Read the model definition and answer for the solid it produces. Units are mm, in the model's axes. Face numbers are marked on the shaded views. Give positions to 0.01 mm unless a question says otherwise; leave off trailing zeros. Order: outer loops, then holes, each group sorted by start corner. A loop starts at its lowest first (then second) coordinate and runs counter-clockwise, first axis right, second up. Notation, with made-up numbers: (80, 78.5) - (133, 78.5) arc R12 ccw to (133, 87.5) - close; hole circle Ø2 at (74.25, 38.5). An arc over 180 degrees is marked (long way). Write each question's results on one line, items separated by ' | '. Start each with the question number.
Q1. Flat-ended cylindrical pins translate along their axes: P1, Ø2.5, axis at x = 42, y = 40.5, coming from the +Z side; P2, Ø6, axis at x = -41, y = 41, coming from the +Z side; P3, Ø10.5, axis at x = 41, y = -41, coming from the +Z side; P4, Ø12, axis at x = -57.98, y = 0, coming from the -Z side. Find the tip coordinate at first contact, or state that the pin passes through.
Q2. Find section B-B on z = 4.25. Give the vertices of the cut face in (x, y).
Q3. Find the intervals of material crossed by line 1 along Y through (x, z) = (0, 8); line 2 along Y through (x, z) = (39, 15); line 3 along Z through (x, y) = (20, 31), in increasing order. Write a range as from..to.
Q4. For a pull along Y with two mould halves and no side action, classify the marked faces 1 and 2 as +Y half, -Y half, draft (parallel to the pull), parting line (faces both ways), or undercut.
Q5. Find section C-C on x = 115. Give the vertices of the cut face in (y, z).
Q6. Find section D-D on y = 83. Give the vertices of the cut face in (x, z).
Q7. Find section A-A on y = 0. Give the vertices of the cut face in (x, z), and give its area (3 significant figures).
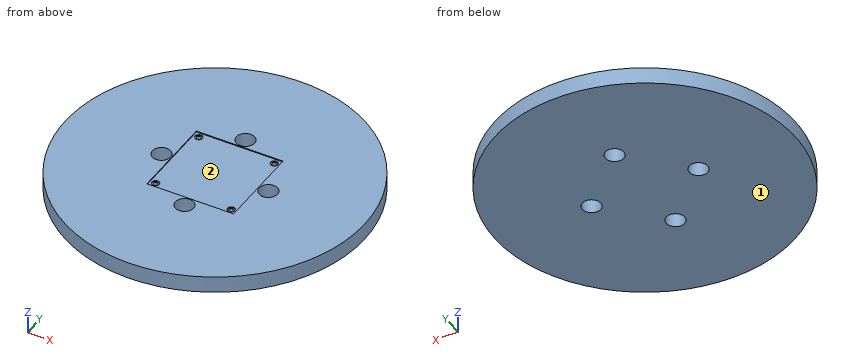
from build123d import *

# Parameters (mm, degrees)
SKETCH003_R      = 162.0844056183
PAD002_DEPTH     = 18
SKETCH009_W      = 94
SKETCH009_H      = 94
POCKET002_DEPTH  = 1
HOLE_D           = 5
HOLE_DEPTH       = 10
HOLE_CBORE_D     = 8
HOLE_CBORE_DEPTH = 1
SKETCH011_R      = 10
POCKET003_DEPTH  = 18.001


with BuildPart() as part:
    # Sketch003 → Pad002 (new body)
    with BuildSketch(Plane.XY):
        Circle(SKETCH003_R)
    extrude(amount=PAD002_DEPTH)

    # Sketch009 (on Face3 of Pad002) → Pocket002 (cut)
    with BuildSketch(Plane.XY.offset(18)):
        Rectangle(SKETCH009_W, SKETCH009_H)
    extrude(amount=-POCKET002_DEPTH, mode=Mode.SUBTRACT)

    # Hole
    with Locations(Plane.XY.offset(17)):
        with Locations((-41, 41), (41, 41), (-41, -41), (41, -41)):
            CounterBoreHole(HOLE_D / 2, HOLE_CBORE_D / 2, HOLE_CBORE_DEPTH, depth=HOLE_DEPTH)

    # Sketch011 (on Face3 of Hole) → Pocket003 (cut, through all)
    with BuildSketch(Plane.XY.offset(18)):
        with Locations((-57.9827560573, 0)):
            Circle(SKETCH011_R)
        with Locations((0, 57.9827560573)):
            Circle(SKETCH011_R)
        with Locations((57.9827560573, 0)):
            Circle(SKETCH011_R)
        with Locations((0, -57.9827560573)):
            Circle(SKETCH011_R)
    extrude(amount=-POCKET003_DEPTH, mode=Mode.SUBTRACT)


with BuildPart() as part_1:
    # Clone004 placement: moved
    add(part.part.moved(Location((0, 0, -24))))


with BuildPart() as part_2:
    # Clone015 placement: moved
    add(part_1.part.moved(Location((0, 0, 24))))


solid = part_2.part
Working result:
1) P1: z = 7 | P2: z = 16 | P3: z = 17 | P4: through
2) outline: circle Ø324.17 at (0, 0); hole circle Ø20 at (-57.98, 0); hole circle Ø20 at (0, -57.98); hole circle Ø20 at (0, 57.98); hole circle Ø20 at (57.98, 0)
3) line 1: -162.08..-67.98, -47.98..47.98, 67.98..162.08 | line 2: -157.32..-42.5, -39.5..39.5, 42.5..157.32 | line 3: 0..17
4) face 1: draft | face 2: undercut
5) outline: (-114.22, 0) - (114.22, 0) - (114.22, 18) - (-114.22, 18) - close
6) outline: (-139.22, 0) - (139.22, 0) - (139.22, 18) - (-139.22, 18) - close
7) outline: (-162.08, 0) - (-67.98, 0) - (-67.98, 18) - (-162.08, 18) - close; (-47.98, 0) - (47.98, 0) - (47.98, 18) - (47, 18) - (47, 17) - (-47, 17) - (-47, 18) - (-47.98, 18) - close; (67.98, 0) - (162.08, 0) - (162.08, 18) - (67.98, 18) - close | area: 5,020 mm²
